Autodesk Inventor part; units mm, degrees
ref_plane "Plano de trabajo2" through (0, 2.3, 0) normal (0, 1, 0) x (1, 0, 0)
ref_plane "YZ Plane" through (0, 0, 0) normal (1, 0, 0) x (0, 1, 0)
ref_plane "XZ Plane" through (0, 0, 0) normal (0, 1, 0) x (-1, 0, 0)
sketch "Boceto6" plane through (0, 0, 0) normal (0, 1, 0) x (-1, 0, 0)
  line L0 (0, 0) -> (8.94, 0)
  line L1 (8.94, 0) -> (8.94, -6.196)
  line L2 (8.94, -6.196) -> (0, -6.196)
  line L3 (0, -6.196) -> (0, 0)
  arc A0 (0.25, -0.1) -> (0.25, -0.4) centre (0.25, -0.25) ccw
  arc A1 (0.35, -0.4) -> (0.35, -0.1) centre (0.35, -0.25) ccw
  line L4 (0.25, -0.4) -> (0.35, -0.4)
  line L5 (0.25, -0.1) -> (0.35, -0.1)
  arc A2 (8.59, -0.1) -> (8.59, -0.4) centre (8.59, -0.25) ccw
  arc A3 (8.69, -0.4) -> (8.69, -0.1) centre (8.69, -0.25) ccw
  line L6 (8.59, -0.4) -> (8.69, -0.4)
  line L7 (8.59, -0.1) -> (8.69, -0.1)
  arc A4 (0.25, -5.796) -> (0.25, -6.096) centre (0.25, -5.946) ccw
  arc A5 (0.35, -6.096) -> (0.35, -5.796) centre (0.35, -5.946) ccw
  line L8 (0.25, -6.096) -> (0.35, -6.096)
  line L9 (0.25, -5.796) -> (0.35, -5.796)
  arc A6 (8.59, -5.796) -> (8.59, -6.096) centre (8.59, -5.946) ccw
  arc A7 (8.69, -6.096) -> (8.69, -5.796) centre (8.69, -5.946) ccw
  line L10 (8.59, -6.096) -> (8.69, -6.096)
  line L11 (8.59, -5.796) -> (8.69, -5.796)
extrude "Extrusión4" add sketch "Boceto6" along normal blind 0.6
sketch "Boceto7" plane through (0, 0.6, 0) normal (0, 1, 0) x (1, 0, 0)
  line L0 (-8.59, 5.796) -> (-8.69, 5.796)
  arc A0 (-8.69, 6.096) -> (-8.69, 5.796) centre (-8.69, 5.946) ccw
  line L1 (-8.69, 6.096) -> (-8.59, 6.096)
  arc A1 (-8.59, 5.796) -> (-8.59, 6.096) centre (-8.59, 5.946) ccw
  line L2 (-0.25, 5.796) -> (-0.35, 5.796)
  arc A2 (-0.35, 6.096) -> (-0.35, 5.796) centre (-0.35, 5.946) ccw
  line L3 (-0.35, 6.096) -> (-0.25, 6.096)
  arc A3 (-0.25, 5.796) -> (-0.25, 6.096) centre (-0.25, 5.946) ccw
  line L4 (-8.59, 0.1) -> (-8.69, 0.1)
  arc A4 (-8.69, 0.4) -> (-8.69, 0.1) centre (-8.69, 0.25) ccw
  line L5 (-8.69, 0.4) -> (-8.59, 0.4)
  arc A5 (-8.59, 0.1) -> (-8.59, 0.4) centre (-8.59, 0.25) ccw
  line L6 (-0.25, 0.1) -> (-0.35, 0.1)
  arc A6 (-0.35, 0.4) -> (-0.35, 0.1) centre (-0.35, 0.25) ccw
  line L7 (-0.35, 0.4) -> (-0.25, 0.4)
  arc A7 (-0.25, 0.1) -> (-0.25, 0.4) centre (-0.25, 0.25) ccw
  line L8 (-8.94, 0) -> (0, 0)
  line L9 (0, 0) -> (0, 6.196)
  line L10 (0, 6.196) -> (-8.94, 6.196)
  line L11 (-8.94, 6.196) -> (-8.94, 0)
  line L12 (-8.94, 6.196) -> (0, 6.196)
  line L13 (0, 0) -> (0, 6.196)
  line L14 (-0.8, 5.546) -> (-0.8, 0.65)
  line L15 (-0.8, 0.65) -> (-8.14, 0.65)
  line L16 (-8.14, 0.65) -> (-8.14, 5.546)
  line L17 (-8.14, 5.546) -> (-0.8, 5.546)
extrude "Extrusión5" cut sketch "Boceto7" against normal blind 0.4
ref_plane "Plano de trabajo2" through (0, 2.3, 0) normal (0, 1, 0) x (1, 0, 0)
sketch "Boceto9" plane through (0, 2.3, 0) normal (0, 1, 0) x (1, 0, 0)
  line L0 (-8.4305, 5.546) -> (-0.2383, 5.546) construction
  line L1 (-0.2383, 5.546) -> (-0.2383, 0.5947) construction
  line L2 (-0.2383, 0.5947) -> (-8.4305, 0.5947) construction
  line L3 (-8.4305, 0.5947) -> (-8.4305, 5.546) construction
  line L4 (-0.8, 5.546) -> (-8.14, 5.546)
  line L5 (-8.14, 5.546) -> (-8.14, 0.65)
  line L6 (-8.14, 0.65) -> (-0.8, 0.65)
  line L7 (-0.8, 0.65) -> (-0.8, 5.546)
  point P0 (0, 0)
decal "Calcomanía1"
properties part number "screen"
The listing builds one solid part. Answer for the finished solid, in the listing's coordinates (mm). Coordinates: 2 decimals unless noted, no trailing zeros. Write each loop counter-clockwise with the first axis right and the second up, starting at its lowest first coordinate (ties: lowest second). Pieces come first, ordered by that corner, then holes. Notation, with made-up numbers: M 5.25,11 L 21.25,11 A20 ccw 21.25,18 Z; hole C -20.75,-39 d10. An arc over 180 degrees is marked long. Use a Markdown table: item, result. Add a question column.
1. Section A-A (z = -0.25) is taken. Give the vertices of the cut face in (x, y), plus the area to 3 significant figures.
2. Straight lines are drawn through the part: line 1 along Z through (x, y) = (-3, 0.5); line 2 along Y through (x, z) = (-8.25, -4.5); line 3 along X through (y, z) = (0.35, -1.5). For each, find the intervals that lie inside material, in ascending order. Write a range as [from, to].
3. Section B-B (z = -2.5) is taken. Give the vertices of the cut face in (x, y).
4. Section D-D (y = 0.45) is taken. Give the vertices of the cut face in (x, z), plus the area to 3 significant figures.
5. Section C-C (x = -2) is taken. Give the vertices of the cut face in (y, z), plus the area to 3 significant figures.
Data:
| question | item | result |
|---|---|---|
| 1 | outline | M -8.94,0 L -8.84,0 L -8.84,0.2 L -8.94,0.2 Z; M -8.44,0 L -0.5,0 L -0.5,0.2 L -8.44,0.2 Z; M -0.1,0 L 0,0 L 0,0.2 L -0.1,0.2 Z |
| 1 | area | 1.63 mm2 |
| 2 | line 1 | z = [-5.55, -0.65] |
| 2 | line 2 | y = [0, 0.2] |
| 2 | line 3 | x = [-8.14, -0.8] |
| 3 | outline | M -8.94,0 L 0,0 L 0,0.2 L -0.8,0.2 L -0.8,0.6 L -8.14,0.6 L -8.14,0.2 L -8.94,0.2 Z |
| 4 | outline | M -8.14,-5.55 L -0.8,-5.55 L -0.8,-0.65 L -8.14,-0.65 Z |
| 4 | area | 35.9 mm2 |
| 5 | outline | M 0,-6.2 L 0.2,-6.2 L 0.2,-5.55 L 0.6,-5.55 L 0.6,-0.65 L 0.2,-0.65 L 0.2,0 L 0,0 Z |
| 5 | area | 3.20 mm2 |
